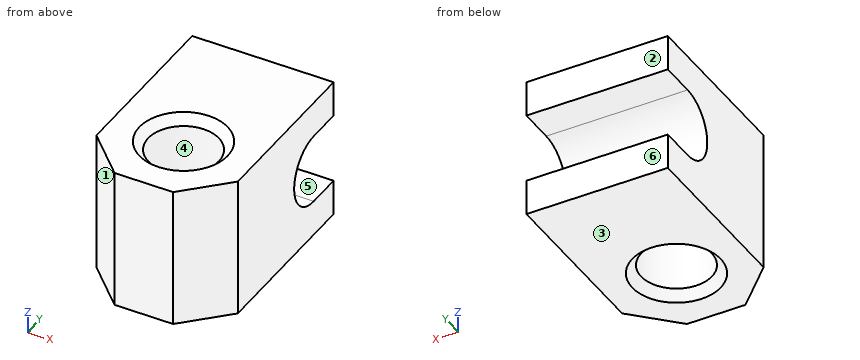
from build123d import *

# Parameters (mm, degrees)
F0_R          = 4
F1_DEPTH      = 8
F3_DEPTH      = 8.001
F3_DEPTH_BACK = 8.001
F4_SIZE       = 1


with BuildPart() as f1:
    # F0 (on Top) → F1 (new body, symmetric)
    with BuildSketch(Plane.XY):
        Polygon((-8, 16), (-8, 0), (-8, -3.313708499), (-3.313708499, -8), (3.313708499, -8), (8, -3.313708499), (8, 0), (8, 16), align=None)
        Circle(F0_R, mode=Mode.SUBTRACT)
    extrude(amount=F1_DEPTH, both=True)

    # F2 (on Right) → F3 (cut, two sides)
    with BuildSketch(Plane.YZ) as f3_sk:
        with BuildLine():
            Line((16, 3.95), (12, 3.95))
            ThreePointArc((12, 3.95), (8.05, 0), (12, -3.95))
            Line((12, -3.95), (16, -3.95))
            Line((16, -3.95), (16, 3.95))
        make_face()
    extrude(amount=-F3_DEPTH, mode=Mode.SUBTRACT)
    extrude(f3_sk.sketch, amount=F3_DEPTH_BACK, mode=Mode.SUBTRACT)

    # F4
    f4_edges = [f1.edges().sort_by_distance(p)[0] for p in [
        (-4, 0, 8),
        (-4, 0, -8),
    ]]
    chamfer(f4_edges, length=F4_SIZE)


solid = f1.part
Check sheet for the modelled part. Datum: model origin and axes. Units: mm. Face numbers are marked on the shaded views. A direction names the side the tool comes from. Round coordinates to 2 decimals unless told otherwise and drop trailing zeros. Loops run counter-clockwise (first coordinate to the right, second up) from the corner with the lowest first, then second, coordinate; pieces in that order, holes last.
1. Sectioned sample at A-A on y = 12.5. Record the boundary of the cut face in (x, z), and give its area (3 significant figures).
2. Scan lines: probe 1 along Z at (x, y) = (4.5, 12); probe 2 along Y at (x, z) = (0, 1.5); probe 3 along Y at (x, z) = (0, 2.25). Record each from-to range of solid material in increasing order.
3. Gauge pin test, flat ends, axial feed: pin 1 Ø4 at (y, z) = (-5.5, 4.5) entering from -X; pin 2 Ø2 at (x, z) = (-3, -1.5) entering from +Y; pin 3 Ø2 at (x, y) = (3, -2.5) entering from +Z. Record the tip position at first contact, or that the pin passes through.
4. Sectioned sample at C-C on z = 0. Record the boundary of the cut face in (x, y).
5. Mould release check, pull along Y, two halves, no side actions. Record for the marked faces 1, 2, 3 and 4: released by +Y, released by -Y, zero draft, split by the parting line, or undercut.
6. Sectioned sample at B-B on x = 0. Record the boundary of the cut face in (y, z).
7. Sectioned sample at D-D on z = 6. Record the boundary of the cut face in (x, y), and give its area (3 significant figures).
8. Set-up check for the marked faces 5 and 6: record each of +Z, -Z, +X, -X, +Y, -Y from which the full face is reachable in a straight line by a thin tool's end or side.
Recorded:
1. outline: (-8, -8) - (8, -8) - (8, -3.95) - (-8, -3.95) - close; (-8, 3.95) - (8, 3.95) - (8, 8) - (-8, 8) - close
1. area: 130 mm2
2. probe 1: z = -8 to -3.95, 3.95 to 8
2. probe 2: y = -8 to -4, 4 to 8.35
2. probe 3: y = -8 to -4, 4 to 8.75
3. pin 1: stops at x = -7.81
3. pin 2: stops at y = 8.94
3. pin 3: stops at z = 7.91
4. outline: (-8, -3.31) - (-3.31, -8) - (3.31, -8) - (8, -3.31) - (8, 8.05) - (-8, 8.05) - close; hole circle Ø8 at (0, 0)
5. face 1: released by -Y
5. face 2: released by +Y
5. face 3: zero draft
5. face 4: undercut
6. outline: (-8, -8) - (-5, -8) - (-4, -7) - (-4, 7) - (-5, 8) - (-8, 8) - close; (4, -7) - (5, -8) - (16, -8) - (16, -3.95) - (12, -3.95) arc R3.95 cw to (12, 3.95) - (16, 3.95) - (16, 8) - (5, 8) - (4, 7) - close
7. outline: (-8, -3.31) - (-3.31, -8) - (3.31, -8) - (8, -3.31) - (8, 16) - (-8, 16) - close; hole circle Ø8 at (0, 0)
7. area: 312 mm2
8. face 5: +X, -X, +Y
8. face 6: +Z, -Z, +X, -X, +Y
